Source: CAD feature listing. Evaluate the final solid. Frame: model axes, mm. A direction names the side the tool comes from. Give positions to 0.01 mm unless a question says otherwise; leave off trailing zeros. Loops run counter-clockwise (first coordinate to the right, second up) from the corner with the lowest first, then second, coordinate; pieces in that order, holes last. Notation, with made-up numbers: (26, -9) -> (51, -9) arc R23 cw to (51, 22) -> close; hole circle Ø1 at (-24.5, 7). An arc over 180 degrees is marked (long way). Return JSON: item names as keys, results as strings. Group by question number.
(1) Access query for faces 1 (the face through (2, 2, 0)), 2 (the face through (-6, 0, 8)). Directions: +Z, -Z, +X, -X, +Y, -Y. A direction counts if a zero-diameter tool reaches every point of the face in a straight line with its end or side. Return the directions, or none.
(2) Cut plane A-A on y = 0. Return loops of the section in (x, z), then the cut area to 4 significant figures.
(3) Draft query along X for faces 3 (the face through (8.6, 1, 7)), 4 (the face through (-8.6, 1, 7)), 5 (the face through (0, 6.421, 7)), 6 (the face through (-1.4, 2, 1.5)). Return one class per face: released by +X, released by -X, zero draft, split by the parting line, or undercut.
(4) Cut plane C-C on z = 11. Return loops of the section in (x, y), then the cut area to 3 significant figures.
(5) Pin query (flat end, axial travel): pin 1 (3.5 mm diameter, centred on x = 0, y = 0, fed in from +Z). Return the tip coordinate at first contact, or that it passes through.
(6) Cut plane D-D on y = 2.5. Return loops of the section in (x, z), then the cut area to 3 significant figures.
(7) Cut plane B-B on x = 0. Return loops of the section in (y, z).
(8) Ray query, line 1 (X direction, y = -2.25, z = 10.25); line 2 (Y direction, x = 0, z = 0.6); line 3 (Y direction, x = -3, z = 4.25). Return the intervals inside material, ascending. Write a range as from..to.
```python
from build123d import *

# Parameters (mm, degrees)
F0_W     = 17.2
F0_H     = 11.7
F0_W_2   = 12
F0_H_2   = 6
F1_DEPTH = 15
F2_R     = 1.5
F0_R     = 2.25
F3_DEPTH = 1.5


# Not quite as in the source:
# - a feature names something its author has since deleted; it is built from what else it names


with BuildPart() as f1:
    # F0 (on Top) → F1 (new body)
    with BuildSketch(Plane.XY):
        with Locations((0, 0.571324781)):
            Rectangle(F0_W, F0_H)
        Rectangle(F0_W_2, F0_H_2, mode=Mode.SUBTRACT)
    extrude(amount=F1_DEPTH)

    # F2
    f2_edges = [f1.edges().sort_by_distance(p)[0] for p in [
        (-8.6, 6.421325, 7.5),
        (8.6, 6.421325, 7.5),
        (8.6, -5.278675, 7.5),
        (-8.6, -5.278675, 7.5),
    ]]
    fillet(f2_edges, radius=F2_R)

    # F0 (on Top) → F3 (join)
    with BuildSketch(Plane.XY):
        Rectangle(F0_W_2, F0_H_2)
        Circle(F0_R, mode=Mode.SUBTRACT)
    extrude(amount=F3_DEPTH)


solid = f1.part
```
Answers:
{
 "1": {"face 1": "-Z, +X, -X, +Y, -Y", "face 2": "+Z"},
 "2": {"outline": "(-8.6, 0) -> (-2.25, 0) -> (-2.25, 1.5) -> (-6, 1.5) -> (-6, 15) -> (-8.6, 15) -> close; (2.25, 0) -> (8.6, 0) -> (8.6, 15) -> (6, 15) -> (6, 1.5) -> (2.25, 1.5) -> close", "area": "89.25 mm²"},
 "3": {"face 3": "released by +X", "face 4": "released by -X", "face 5": "zero draft", "face 6": "undercut"},
 "4": {"outline": "(-8.6, -3.78) arc R1.5 ccw to (-7.1, -5.28) -> (7.1, -5.28) arc R1.5 ccw to (8.6, -3.78) -> (8.6, 4.92) arc R1.5 ccw to (7.1, 6.42) -> (-7.1, 6.42) arc R1.5 ccw to (-8.6, 4.92) -> close; hole (-6, -3) -> (6, -3) -> (6, 3) -> (-6, 3) -> close", "area": "127 mm²"},
 "5": {"pin 1": "through"},
 "6": {"outline": "(-8.6, 0) -> (8.6, 0) -> (8.6, 15) -> (6, 15) -> (6, 1.5) -> (-6, 1.5) -> (-6, 15) -> (-8.6, 15) -> close", "area": "96.0 mm²"},
 "7": {"outline": "(-5.28, 0) -> (-2.25, 0) -> (-2.25, 1.5) -> (-3, 1.5) -> (-3, 15) -> (-5.28, 15) -> close; (2.25, 0) -> (6.42, 0) -> (6.42, 15) -> (3, 15) -> (3, 1.5) -> (2.25, 1.5) -> close"},
 "8": {"line 1": "-8.6..-6, 6..8.6", "line 2": "-5.28..-2.25, 2.25..6.42", "line 3": "-5.28..-3, 3..6.42"}
}
